from build123d import *

# Parameters (mm, degrees)
SKETCH1_W             = 60
SKETCH1_H             = 20
BOSS_EXTRUDE1_DEPTH   = 46
SKETCH2_W             = 10
SKETCH2_H             = 8
CUT_EXTRUDE1_DEPTH    = 10
F_3_0MM_DOWEL_HOLE1_D = 3
SKETCH5_W             = 10
SKETCH5_H             = 10
CUT_EXTRUDE2_DEPTH    = 10
M3_CLEARANCE_HOLE1_D  = 3.2


with BuildPart() as part:
    # Sketch1 → Boss-Extrude1 (new body)
    with BuildSketch(Plane(origin=(0, 0, 0), x_dir=(1, 0, 0), z_dir=(0, 1, 0))):
        Rectangle(SKETCH1_W, SKETCH1_H)
    extrude(amount=BOSS_EXTRUDE1_DEPTH)

    # Sketch2 → Cut-Extrude1 (cut)
    with BuildSketch(Plane(origin=(30, 0, 0), x_dir=(0, 0, -1), z_dir=(1, 0, 0))):
        with Locations((5, 23)):
            Rectangle(SKETCH2_W, SKETCH2_H)
    extrude(amount=-CUT_EXTRUDE1_DEPTH, mode=Mode.SUBTRACT)

    # Ø3.0mm Dowel Hole1 (through all)
    with Locations(Plane(origin=(0, 46, 0), x_dir=(1, 0, 0), z_dir=(0, 1, 0))):
        with Locations((-27, 7), (27, 7)):
            Hole(F_3_0MM_DOWEL_HOLE1_D / 2)

    # Sketch5 → Cut-Extrude2 (cut)
    with BuildSketch(Plane.ZY.offset(30)):
        with Locations((-5, 23)):
            Rectangle(SKETCH5_W, SKETCH5_H)
    extrude(amount=-CUT_EXTRUDE2_DEPTH, mode=Mode.SUBTRACT)

    # M3 Clearance Hole1 (through all)
    with Locations(Plane(origin=(0, 46, 0), x_dir=(1, 0, 0), z_dir=(0, 1, 0))):
        with Locations((-25, -5), (0, 5), (25, -5)):
            Hole(M3_CLEARANCE_HOLE1_D / 2)


solid = part.part
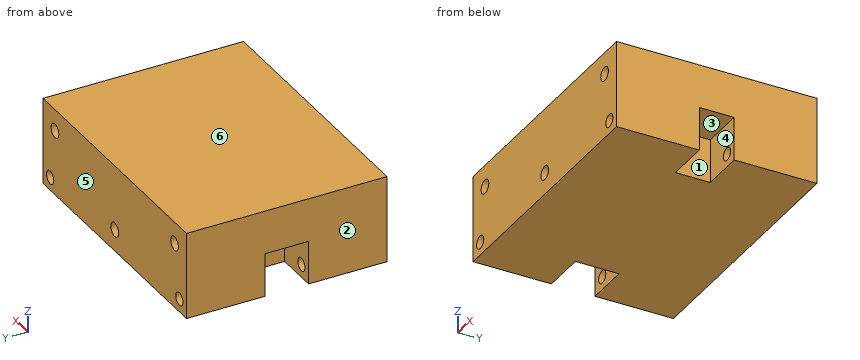
The model under review builds one solid part; all positions refer to its coordinate system, in mm. Face numbers are marked on the shaded views. A direction names the side the tool comes from. Round coordinates to 2 decimals unless told otherwise and drop trailing zeros. Loops run counter-clockwise (first coordinate to the right, second up) from the corner with the lowest first, then second, coordinate; pieces in that order, holes last. Notation, with made-up numbers: (86, -7) -> (127, -7) arc R23 cw to (127, 9) -> close; hole circle Ø1 at (39.5, 29). An arc over 180 degrees is marked (long way). One line per question, with ' | ' between items. Start each with the question number.
Item 1: Machinability: for the marked faces 1 and 2, which of the approach directions +Z, -Z, +X, -X, +Y, -Y give a long, thin tool a straight path to every point of the face, cutting with its end or side? Answer none if there is none.
Item 2: Add section A-A, the plane y = 8.5. Write out the cut boundary in (x, z).
Item 3: Wall thickness on line 1 along X through (y, z) = (41, -7); line 2 along X through (y, z) = (22, 5); line 3 along Y through (x, z) = (25.5, -5.25): over which ranges is each line inside the solid? List them lowest first. Write a range as [from, to].
Item 4: Add section B-B, the plane x = 0. Write out the cut boundary in (y, z), then the cut area to 3 significant figures.
Item 5: For pin 1 (6.5 mm diameter, centred on x = 24, y = 22.5, fed in from -Z); pin 2 (2.5 mm diameter, centred on x = -25, z = 5, fed in from +Y); pin 3 (4 mm diameter, centred on y = 22.5, z = -4.5, fed in from +X); pin 4 (8 mm diameter, centred on y = 22.5, z = -6, fed in from -X), all flat-tipped, find the tip position at first contact; note any pin that passes through.
Item 6: Add section D-D, the plane z = -2.5. Write out the cut boundary in (x, y).
Item 7: Draft analysis for pull direction Y (two halves, no side actions). For the marked faces 3, 4, 5 and 6, state which applies: +Y half, -Y half, draft (parallel to the pull), parting line (faces both ways), or undercut.
Item 8: Add section C-C, the plane y = 25. Write out the cut boundary in (x, z), then the cut area to 3 significant figures.
Return value:
1) face 1: -Z, +X | face 2: +Z, -Z, -X, +Y, -Y
2) outline: (-30, -10) -> (30, -10) -> (30, 10) -> (-30, 10) -> close; hole circle Ø3 at (-27, -7); hole circle Ø3.2 at (-25, 5); hole circle Ø3.2 at (0, -5); hole circle Ø3.2 at (25, 5); hole circle Ø3 at (27, -7)
3) line 1: x = [-30, -28.5], [-25.5, 25.5], [28.5, 30] | line 2: x = [-30, -26.6], [-23.4, 23.4], [26.6, 30] | line 3: y = [0, 19], [27, 46]
4) outline: (0, -10) -> (46, -10) -> (46, -6.6) -> (0, -6.6) -> close; (0, -3.4) -> (46, -3.4) -> (46, 10) -> (0, 10) -> close | area: 773 mm2
5) pin 1: stops at z = 0 | pin 2: passes through | pin 3: stops at x = 20 | pin 4: stops at x = -20
6) outline: (-30, 0) -> (30, 0) -> (30, 19) -> (20, 19) -> (20, 27) -> (30, 27) -> (30, 46) -> (-30, 46) -> (-30, 28) -> (-20, 28) -> (-20, 18) -> (-30, 18) -> close
7) face 3: undercut | face 4: undercut | face 5: +Y half | face 6: draft
8) outline: (-30, 0) -> (-20, 0) -> (-20, -10) -> (20, -10) -> (20, 0) -> (30, 0) -> (30, 10) -> (-30, 10) -> close; hole circle Ø3.2 at (-25, 5); hole circle Ø3.2 at (0, -5); hole circle Ø3.2 at (25, 5) | area: 976 mm2
